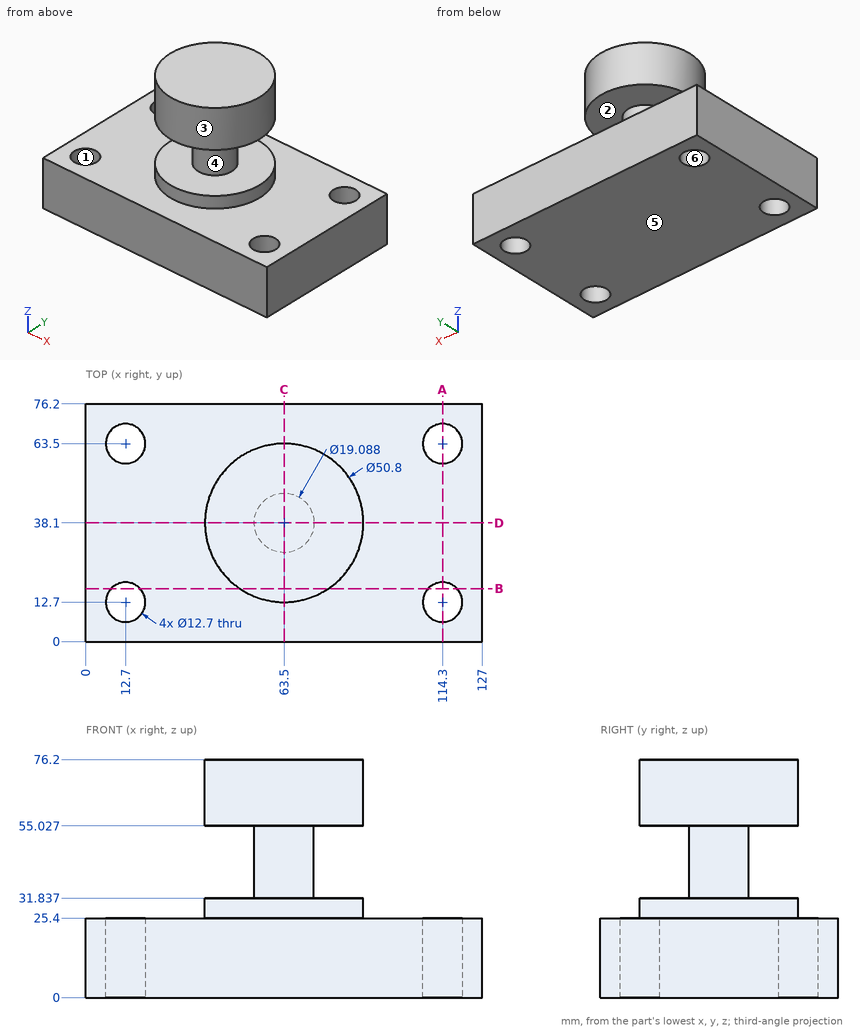
Verification items for this drawing (mm, ordinates from the low corner). A direction names the side the tool comes from. Coordinates: 2 decimals unless noted, no trailing zeros. Order: outer loops, then holes, each group sorted by start corner. A loop starts at its lowest first (then second) coordinate and runs counter-clockwise, first axis right, second up. Notation, with made-up numbers: (83, 57.5) - (89, 57.5) arc R22 ccw to (89, 83.5) - close; hole circle Ø6 at (47.25, 17.25). An arc over 180 degrees is marked (long way). Use one line per item in the form item = value.
1. Section check A-A (x = 114.3). Record the boundary of the cut face in (y, z), then the cut area to 3 significant figures.
Here are the results:
outline = (0, 0) - (6.35, 0) - (6.35, 25.4) - (0, 25.4) - close; (19.05, 0) - (57.15, 0) - (57.15, 25.4) - (19.05, 25.4) - close; (69.85, 0) - (76.2, 0) - (76.2, 25.4) - (69.85, 25.4) - close
area = 1,290 mm²
2. Draft check along X on the marked faces 4, 5 and 6. Enter one of: pulls with the +X half, pulls with the -X half, needs draft (parallel to the pull), parting line crosses it, or undercut.
Here are the results:
face_4 = parting line crosses it
face_5 = needs draft
face_6 = undercut
3. Gauge pin test, flat ends, axial feed: pin 1 (4 mm diameter, centred on y = 31.5, z = 32, fed in from +X); pin 2 (10 mm diameter, centred on x = 12.7, y = 63.5, fed in from +Z); pin 3 (5 mm diameter, centred on x = 28, y = 59.5, fed in from +Z); pin 4 (4 mm diameter, centred on y = 43.5, z = 54, fed in from -X). Record the tip position at first contact, or that the pin passes through.
Here are the results:
pin_1 = 88.48
pin_2 = through
pin_3 = 25.4
pin_4 = 38.37
4. Section check B-B (y = 17). Record the boundary of the cut face in (x, z), then the cut area to 3 significant figures.
Here are the results:
outline = (0, 0) - (8.03, 0) - (8.03, 25.4) - (0, 25.4) - close; (17.37, 0) - (109.63, 0) - (109.63, 25.4) - (77.64, 25.4) - (77.64, 31.84) - (49.36, 31.84) - (49.36, 25.4) - (17.37, 25.4) - close; (49.36, 55.03) - (77.64, 55.03) - (77.64, 76.2) - (49.36, 76.2) - close; (118.97, 0) - (127, 0) - (127, 25.4) - (118.97, 25.4) - close
area = 3,530 mm²
5. Scan lines: line 1 (Y direction, x = 114.3, z = 16.75); line 2 (X direction, y = 12, z = 16); line 3 (Z direction, x = 76, y = 54). Record each from-to range of solid material in increasing order.
Here are the results:
line_1 = 0 to 6.35, 19.05 to 57.15, 69.85 to 76.2
line_2 = 0 to 6.39, 19.01 to 107.99, 120.61 to 127
line_3 = 0 to 31.84, 55.03 to 76.2
6. Access from +Z, -Z, +X, -X, +Y, -Y to the whole of each face (thin tool, end or side, straight path). Record for the marked faces 1, 2 and 3.
Here are the results:
face_1 = +Z, -Z
face_2 = none
face_3 = +Z
7. Section check C-C (x = 63.5). Record the boundary of the cut face in (y, z).
Here are the results:
outline = (0, 0) - (76.2, 0) - (76.2, 25.4) - (63.5, 25.4) - (63.5, 31.84) - (47.64, 31.84) - (47.64, 55.03) - (63.5, 55.03) - (63.5, 76.2) - (12.7, 76.2) - (12.7, 55.03) - (28.56, 55.03) - (28.56, 31.84) - (12.7, 31.84) - (12.7, 25.4) - (0, 25.4) - close
8. Section check D-D (y = 38.1). Record the boundary of the cut face in (x, z), then the cut area to 3 significant figures.
Here are the results:
outline = (0, 0) - (127, 0) - (127, 25.4) - (88.9, 25.4) - (88.9, 31.84) - (73.04, 31.84) - (73.04, 55.03) - (88.9, 55.03) - (88.9, 76.2) - (38.1, 76.2) - (38.1, 55.03) - (53.96, 55.03) - (53.96, 31.84) - (38.1, 31.84) - (38.1, 25.4) - (0, 25.4) - close
area = 5,070 mm²
